Read the model definition and answer for the solid it produces. Units are mm, in the model's axes. Coordinates: 2 decimals unless noted, no trailing zeros. Write each loop counter-clockwise with the first axis right and the second up, starting at its lowest first coordinate (ties: lowest second). Pieces come first, ordered by that corner, then holes. Notation, with made-up numbers: (-8, -38.5) -> (-4, -38.5) arc R22 cw to (-4, -1.5) -> close; hole circle Ø6 at (75, 41). An arc over 180 degrees is marked (long way). Use CSV: the item, a comma, the result in double quotes. Start each with the question number.
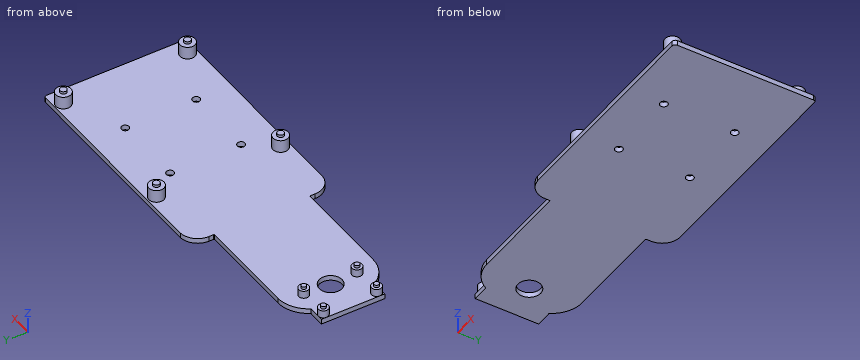
from build123d import *

# Parameters (mm, degrees)
SKETCH_R                  = 1.4
SKETCH_R_2                = 1.5
PAD_DEPTH                 = 2
SKETCH002_R               = 6.353363
PAD002_DEPTH              = 2
CYLINDER022_R             = 1.3
CYLINDER022_DEPTH         = 8
CYLINDER021_R             = 3
CYLINDER021_DEPTH         = 7
CYLINDER019_R             = 1.3
CYLINDER019_DEPTH         = 8
CYLINDER020_R             = 3
CYLINDER020_DEPTH         = 7
CYLINDER011_R             = 1.3
CYLINDER011_DEPTH         = 8
CYLINDER008_R             = 3
CYLINDER008_DEPTH         = 7
CYLINDER013_R             = 1.3
CYLINDER013_DEPTH         = 8
CYLINDER012_R             = 3
CYLINDER012_DEPTH         = 7
CYLINDER006_R             = 1
CYLINDER006_DEPTH         = 6
CYLINDER005_R             = 2
CYLINDER005_DEPTH         = 5
CYLINDER007_R             = 1
CYLINDER007_DEPTH         = 6
CYLINDER004_R             = 2
CYLINDER004_DEPTH         = 5
CYLINDER003_R             = 1
CYLINDER003_DEPTH         = 6
CYLINDER002_R             = 2
CYLINDER002_DEPTH         = 5
CYLINDER001_R             = 1
CYLINDER001_DEPTH         = 6
CYLINDER_R                = 2
CYLINDER_DEPTH            = 5
SKETCH001_W               = 25
SKETCH001_H               = 23.8
SKETCH001_R               = 1
SKETCH001_R_2             = 4.5
PAD001_DEPTH              = 2
FUSION006_PLACEMENT_ANGLE = 90


with BuildPart() as opa:
    # Sketch → Pad (new body)
    with BuildSketch(Plane.XY):
        with BuildLine():
            Line((-42.5, 28), (41.5, 28))
            ThreePointArc((42.5, 27), (42.207107, 27.707107), (41.5, 28))
            Line((42.5, 27), (42.5, -26.687649))
            ThreePointArc((41.187649, -28), (42.115621, -27.615621), (42.5, -26.687649))
            Line((41.187649, -28), (-42.5, -28))
            Line((-42.5, -28), (-42.5, 28))
        make_face()
        with Locations((-22, 24.5)):
            Circle(SKETCH_R, mode=Mode.SUBTRACT)
        with Locations((36, 24.5)):
            Circle(SKETCH_R, mode=Mode.SUBTRACT)
        with Locations((-14, 14)):
            Circle(SKETCH_R_2, mode=Mode.SUBTRACT)
        with Locations((14, 14)):
            Circle(SKETCH_R_2, mode=Mode.SUBTRACT)
        with Locations((-14, -14)):
            Circle(SKETCH_R_2, mode=Mode.SUBTRACT)
        with Locations((14, -14)):
            Circle(SKETCH_R_2, mode=Mode.SUBTRACT)
        with Locations((-22, -24.5)):
            Circle(SKETCH_R, mode=Mode.SUBTRACT)
        with Locations((36, -24.5)):
            Circle(SKETCH_R, mode=Mode.SUBTRACT)
    extrude(amount=PAD_DEPTH)


with BuildPart() as body002:
    # Sketch002 → Pad002 (new body)
    with BuildSketch(Plane.XY):
        with BuildLine():
            Line((-49.402144, 18.840823), (-88.680573, 18.840823))
            ThreePointArc((-88.680573, 18.840823), (-97.237161, 15.296568), (-100.781416, 6.73998))
            Line((-100.781416, 6.73998), (-100.781416, -6.73998))
            ThreePointArc((-100.781416, -6.73998), (-97.237161, -15.296568), (-88.680573, -18.840823))
            Line((-88.680573, -18.840823), (-49.411004, -18.840823))
            ThreePointArc((-49.109699, -19.142128), (-49.197949, -18.929073), (-49.411004, -18.840823))
            Line((-49.109699, -19.142128), (-49.109699, -20.971369))
            ThreePointArc((-49.109699, -20.971369), (-47.197032, -25.790971), (-42.5, -27.987504))
            Line((-42.5, -27.987504), (-42.5, 27.983629))
            ThreePointArc((-42.5, 27.983629), (-47.200179, 25.749755), (-49.109699, 20.908721))
            Line((-49.109699, 20.908721), (-49.109699, 19.133268))
            ThreePointArc((-49.402144, 18.840823), (-49.195354, 18.926478), (-49.109699, 19.133268))
        make_face()
        with Locations((-91.871376, 0)):
            Circle(SKETCH002_R, mode=Mode.SUBTRACT)
    extrude(amount=PAD002_DEPTH)


with BuildPart() as cylinder022:
    # Cylinder022 → Cylinder022 (new body)
    with BuildSketch(Plane.XY):
        Circle(CYLINDER022_R)
    extrude(amount=CYLINDER022_DEPTH)


with BuildPart() as fusion022:
    # Cylinder021 → Cylinder021 (new body)
    with BuildSketch(Plane.XY):
        Circle(CYLINDER021_R)
    extrude(amount=CYLINDER021_DEPTH)

    # Fusion022: union Cylinder022
    add(cylinder022.part)


with BuildPart() as fusion022_1:
    # Fusion022 placement: moved
    add(fusion022.part.moved(Location((-39, 24.5, 0))))


with BuildPart() as cylinder019:
    # Cylinder019 → Cylinder019 (new body)
    with BuildSketch(Plane.XY):
        Circle(CYLINDER019_R)
    extrude(amount=CYLINDER019_DEPTH)


with BuildPart() as fusion024:
    # Cylinder020 → Cylinder020 (new body)
    with BuildSketch(Plane.XY):
        Circle(CYLINDER020_R)
    extrude(amount=CYLINDER020_DEPTH)

    # Fusion023: union Cylinder019
    add(cylinder019.part)


with BuildPart() as fusion024_1:
    # Fusion023 placement: moved
    add(fusion024.part.moved(Location((-39, -24.5, 0))))

    # Fusion024: union Fusion022
    add(fusion022_1.part)


with BuildPart() as fusion024_2:
    # Fusion024 placement: moved
    add(fusion024_1.part.moved(Location((58, 0, 0))))


with BuildPart() as cylinder011:
    # Cylinder011 → Cylinder011 (new body)
    with BuildSketch(Plane.XY):
        Circle(CYLINDER011_R)
    extrude(amount=CYLINDER011_DEPTH)


with BuildPart() as fusion007:
    # Cylinder008 → Cylinder008 (new body)
    with BuildSketch(Plane.XY):
        Circle(CYLINDER008_R)
    extrude(amount=CYLINDER008_DEPTH)

    # Fusion007: union Cylinder011
    add(cylinder011.part)


with BuildPart() as fusion007_1:
    # Fusion007 placement: moved
    add(fusion007.part.moved(Location((-39, 24.5, 0))))


with BuildPart() as cylinder013:
    # Cylinder013 → Cylinder013 (new body)
    with BuildSketch(Plane.XY):
        Circle(CYLINDER013_R)
    extrude(amount=CYLINDER013_DEPTH)


with BuildPart() as fusion025:
    # Cylinder012 → Cylinder012 (new body)
    with BuildSketch(Plane.XY):
        Circle(CYLINDER012_R)
    extrude(amount=CYLINDER012_DEPTH)

    # Fusion008: union Cylinder013
    add(cylinder013.part)


with BuildPart() as fusion025_1:
    # Fusion008 placement: moved
    add(fusion025.part.moved(Location((-39, -24.5, 0))))

    # Fusion009: union Fusion007
    add(fusion007_1.part)

    # Fusion025: union Fusion024
    add(fusion024_2.part)


with BuildPart() as fusion025_2:
    # Fusion025 placement: moved
    add(fusion025_1.part.moved(Location((17, 0, 0))))


with BuildPart() as cylinder006:
    # Cylinder006 → Cylinder006 (new body)
    with BuildSketch(Plane.XY):
        Circle(CYLINDER006_R)
    extrude(amount=CYLINDER006_DEPTH)


with BuildPart() as fusion004:
    # Cylinder005 → Cylinder005 (new body)
    with BuildSketch(Plane.XY):
        Circle(CYLINDER005_R)
    extrude(amount=CYLINDER005_DEPTH)

    # Fusion004: union Cylinder006
    add(cylinder006.part)


with BuildPart() as fusion004_1:
    # Fusion004 placement: moved
    add(fusion004.part.moved(Location((10.5, -2.3, 0))))


with BuildPart() as cylinder007:
    # Cylinder007 → Cylinder007 (new body)
    with BuildSketch(Plane.XY):
        Circle(CYLINDER007_R)
    extrude(amount=CYLINDER007_DEPTH)


with BuildPart() as fusion005:
    # Cylinder004 → Cylinder004 (new body)
    with BuildSketch(Plane.XY):
        Circle(CYLINDER004_R)
    extrude(amount=CYLINDER004_DEPTH)

    # Fusion003: union Cylinder007
    add(cylinder007.part)


with BuildPart() as fusion005_1:
    # Fusion003 placement: moved
    add(fusion005.part.moved(Location((-10.5, -2.3, 0))))

    # Fusion005: union Fusion004
    add(fusion004_1.part)


with BuildPart() as fusion005_2:
    # Fusion005 placement: moved
    add(fusion005_1.part.moved(Location((0, 12.2, 0))))


with BuildPart() as cylinder003:
    # Cylinder003 → Cylinder003 (new body)
    with BuildSketch(Plane.XY):
        Circle(CYLINDER003_R)
    extrude(amount=CYLINDER003_DEPTH)


with BuildPart() as fusion001:
    # Cylinder002 → Cylinder002 (new body)
    with BuildSketch(Plane.XY):
        Circle(CYLINDER002_R)
    extrude(amount=CYLINDER002_DEPTH)

    # Fusion001: union Cylinder003
    add(cylinder003.part)


with BuildPart() as fusion001_1:
    # Fusion001 placement: moved
    add(fusion001.part.moved(Location((10.5, -2.3, 0))))


with BuildPart() as cylinder001:
    # Cylinder001 → Cylinder001 (new body)
    with BuildSketch(Plane.XY):
        Circle(CYLINDER001_R)
    extrude(amount=CYLINDER001_DEPTH)


with BuildPart() as fusion002:
    # Cylinder → Cylinder (new body)
    with BuildSketch(Plane.XY):
        Circle(CYLINDER_R)
    extrude(amount=CYLINDER_DEPTH)

    # Fusion: union Cylinder001
    add(cylinder001.part)


with BuildPart() as fusion002_1:
    # Fusion placement: moved
    add(fusion002.part.moved(Location((-10.5, -2.3, 0))))

    # Fusion002: union Fusion001
    add(fusion001_1.part)


with BuildPart() as obj1:
    # Sketch001 → Pad001 (new body)
    with BuildSketch(Plane.XY):
        Rectangle(SKETCH001_W, SKETCH001_H)
        with Locations((-10.5, 9.9)):
            Circle(SKETCH001_R, mode=Mode.SUBTRACT)
        with Locations((10.5, 9.9)):
            Circle(SKETCH001_R, mode=Mode.SUBTRACT)
        with Locations((-10.5, -2.3)):
            Circle(SKETCH001_R, mode=Mode.SUBTRACT)
        with Locations((10.5, -2.3)):
            Circle(SKETCH001_R, mode=Mode.SUBTRACT)
        with Locations((0, -2.1)):
            Circle(SKETCH001_R_2, mode=Mode.SUBTRACT)
    extrude(amount=PAD001_DEPTH)

    # Fusion006: union Fusion005, Fusion002
    add(fusion005_2.part)
    add(fusion002_1.part)


with BuildPart() as obj1_1:
    # Fusion006 placement: moved
    add(obj1.part.moved(Location((-94, 0, 0))).rotate(Axis((-94, 0, 0), (0, 0, 1)), FUSION006_PLACEMENT_ANGLE))

    # Fusion026: union opa, Body002, Fusion025
    add(opa.part)
    add(body002.part)
    add(fusion025_2.part)


solid = obj1_1.part
1) Find the intervals of material crossed by line 1 along Y through (x, z) = (14, 1.1); line 2 along Y through (x, z) = (36, 5); line 3 along Z through (x, y) = (-14, -2.5), in increasing order.
2) Section D-D, the plane x = -95 is taken. Give the vertices of the cut face in (y, z), plus the area to 3 significant figures.
3) Section A-A, the plane y = 0 is taken. Give the vertices of the cut face in (x, z), plus the area to 3 significant figures.
4) Section B-B, the plane x = -14 is taken. Give the vertices of the cut face in (y, z).
5) Section C-C, the plane x = 36 is taken. Give the vertices of the cut face in (y, z), plus the area to 3 significant figures.
6) Each of these flat-tipped pins is pushed along its axis until it touches: pin 1 (2 mm diameter, centred on x = -91, y = 10, fed in from +Z); pin 2 (1.6 mm diameter, centred on x = -101.5, z = 1.5, fed in from +Y); pin 3 (2 mm diameter, centred on x = -102, z = 0.5, fed in from -Y); pin 4 (1.8 mm diameter, centred on x = -14, y = -14, fed in from -Z). Where does it stop, or does it pass through?
The answers:
1,line 1,"y = -28 to -15.5, -12.5 to 12.5, 15.5 to 28"
1,line 2,"y = -27.5 to -21.5, 21.5 to 27.5"
1,line 3,"z = 0 to 2"
2,outline,"(-17.06, 0) -> (-3.26, 0) -> (-3.26, 2) -> (-17.06, 2) -> close; (3.26, 0) -> (17.06, 0) -> (17.06, 2) -> (3.26, 2) -> close"
2,area,"55.2 mm^2"
3,outline,"(-105.9, 0) -> (-96.4, 0) -> (-96.4, 2) -> (-105.9, 2) -> close; (-87.4, 0) -> (42.5, 0) -> (42.5, 2) -> (-87.4, 2) -> close"
3,area,"279 mm^2"
4,outline,"(-28, 0) -> (-15.5, 0) -> (-15.5, 2) -> (-28, 2) -> close; (-12.5, 0) -> (12.5, 0) -> (12.5, 2) -> (-12.5, 2) -> close; (15.5, 0) -> (28, 0) -> (28, 2) -> (15.5, 2) -> close"
5,outline,"(-28, 0) -> (28, 0) -> (28, 2) -> (27.5, 2) -> (27.5, 7) -> (25.8, 7) -> (25.8, 8) -> (23.2, 8) -> (23.2, 7) -> (21.5, 7) -> (21.5, 2) -> (-21.5, 2) -> (-21.5, 7) -> (-23.2, 7) -> (-23.2, 8) -> (-25.8, 8) -> (-25.8, 7) -> (-27.5, 7) -> (-27.5, 2) -> (-28, 2) -> close"
5,area,"177 mm^2"
6,pin 1,"stops at z = 6"
6,pin 2,"stops at y = 12.5"
6,pin 3,"stops at y = -12.5"
6,pin 4,"passes through"
